Autodesk Inventor part; units mm, degrees
ref_plane "Work Plane1" through (0, 4, 0) normal (0, 1, 0) x (-1, 0, 0)
ref_plane "Work Plane2" through (39, 0, -45) normal (1, 0, 0) x (0, 0, -1)
ref_plane "YZ Plane" through (0, 0, 0) normal (1, 0, 0) x (0, 1, 0)
sketch "Sketch1" plane through (0, 0, 0) normal (0, 1, 0) x (-1, 0, 0)
  line L0 (-10, 0) -> (-63, 0)
  line L1 (-73, -10) -> (-73, -57)
  line L2 (0, -57) -> (0, -10)
  line L3 (-22.5, -57) -> (-22.5, -65)
  line L4 (-22.5, -65) -> (-30, -65)
  line L5 (-30, -65) -> (-30, -57)
  line L6 (-48, -57) -> (-48, -65)
  line L7 (-48, -65) -> (-55.5, -65)
  line L8 (-55.5, -65) -> (-55.5, -57)
  line L9 (-73, -57) -> (-55.5, -57)
  line L10 (-22.5, -57) -> (0, -57)
  line L11 (-37.25, -57) -> (-37.25, -53)
  line L12 (-37.25, -53) -> (-36, -53)
  line L13 (-36, -53) -> (-36, -50)
  line L14 (-36, -50) -> (-37.25, -50)
  line L15 (-37.25, -50) -> (-37.25, -45)
  line L16 (-37.25, -45) -> (-40.75, -45)
  line L17 (-40.75, -45) -> (-40.75, -50)
  line L18 (-40.75, -50) -> (-42, -50)
  line L19 (-42, -50) -> (-42, -53)
  line L20 (-42, -53) -> (-40.75, -53)
  line L21 (-40.75, -53) -> (-40.75, -57)
  line L22 (-48, -57) -> (-40.75, -57)
  line L23 (-37.25, -57) -> (-30, -57)
  arc A0 (0, -10) -> (-10, 0) centre (-10, -10) ccw
  arc A1 (-63, 0) -> (-73, -10) centre (-63, -10) ccw
  line L24 (-5, -17) -> (-10, -17)
  line L25 (-10, -17) -> (-10, -27)
  line L26 (-10, -27) -> (-5, -27)
  line L27 (-5, -27) -> (-5, -17)
  line L28 (-5, -36.5) -> (-10, -36.5)
  line L29 (-10, -36.5) -> (-10, -46.5)
  line L30 (-10, -46.5) -> (-5, -46.5)
  line L31 (-5, -46.5) -> (-5, -36.5)
  line L32 (-63, -17) -> (-68, -17)
  line L33 (-68, -17) -> (-68, -27)
  line L34 (-68, -27) -> (-63, -27)
  line L35 (-63, -27) -> (-63, -17)
  line L36 (-63, -36.5) -> (-68, -36.5)
  line L37 (-68, -36.5) -> (-68, -46.5)
  line L38 (-68, -46.5) -> (-63, -46.5)
  line L39 (-63, -46.5) -> (-63, -36.5)
  line L40 (-39, -45) -> (-39, -65) construction
  point P0 (0, 0)
  point P1 (-73, 0)
  dimension "d0" = 73
  dimension "d1" = 57
  dimension "d2" = 22.5
  dimension "d3" = 7.5
  dimension "d4" = 8
  dimension "d5" = 17.5
  dimension "d6" = 18
  dimension "d7" = 3.5
  dimension "d8" = 6
  dimension "d9" = 4
  dimension "d10" = 3
  dimension "d11" = 5
  dimension "d12" = 10
  dimension "d13" = 5
  dimension "d14" = 10
  dimension "d15" = 5
  dimension "d17" = 9.5
  dimension "d18" = 5
  dimension "d19" = 10.5
extrude "Extrusion1" add sketch "Sketch1" along normal blind 8
sketch "Sketch2" plane through (0, 8, 0) normal (0, 1, 0) x (1, 0, 0)
  line L0 (63, 36.5) -> (63, 46.5) construction
  line L1 (63, 46.5) -> (68, 46.5) construction
  line L2 (68, 46.5) -> (68, 36.5) construction
  line L3 (68, 36.5) -> (63, 36.5) construction
  line L4 (63, 17) -> (63, 27) construction
  line L5 (63, 27) -> (68, 27) construction
  line L6 (68, 27) -> (68, 17) construction
  line L7 (68, 17) -> (63, 17) construction
  line L8 (5, 36.5) -> (5, 46.5) construction
  line L9 (5, 46.5) -> (10, 46.5) construction
  line L10 (10, 46.5) -> (10, 36.5) construction
  line L11 (10, 36.5) -> (5, 36.5) construction
  line L12 (5, 17) -> (5, 27) construction
  line L13 (5, 27) -> (10, 27) construction
  line L14 (10, 27) -> (10, 17) construction
  line L15 (10, 17) -> (5, 17) construction
  line L16 (73, 10) -> (73, 57) construction
  line L17 (73, 57) -> (55.5, 57) construction
  line L18 (55.5, 57) -> (55.5, 65) construction
  line L19 (55.5, 65) -> (48, 65) construction
  line L20 (48, 65) -> (48, 57) construction
  line L21 (48, 57) -> (40.75, 57) construction
  line L22 (40.75, 57) -> (40.75, 53) construction
  line L23 (40.75, 53) -> (42, 53) construction
  line L24 (42, 53) -> (42, 50) construction
  line L25 (42, 50) -> (40.75, 50) construction
  line L26 (40.75, 50) -> (40.75, 45) construction
  line L27 (40.75, 45) -> (37.25, 45) construction
  line L28 (37.25, 45) -> (37.25, 50) construction
  line L29 (37.25, 50) -> (36, 50) construction
  line L30 (36, 50) -> (36, 53) construction
  line L31 (36, 53) -> (37.25, 53) construction
  line L32 (37.25, 53) -> (37.25, 57) construction
  line L33 (37.25, 57) -> (30, 57) construction
  line L34 (30, 57) -> (30, 65) construction
  line L35 (30, 65) -> (22.5, 65) construction
  line L36 (22.5, 65) -> (22.5, 57) construction
  line L37 (22.5, 57) -> (0, 57) construction
  line L38 (0, 57) -> (0, 10) construction
  arc A0 (0, 10) -> (10, 0) centre (10, 10) ccw construction
  line L39 (10, 0) -> (63, 0) construction
  arc A1 (63, 0) -> (73, 10) centre (63, 10) ccw construction
  line L40 (10, 27) -> (5, 27) construction
  line L41 (7.5, 27) -> (7.5, 36.5) construction
  line L42 (5, 36.5) -> (10, 36.5) construction
  line L43 (65.5, 27) -> (65.5, 36.5) construction
  line L44 (68, 36.5) -> (63, 36.5) construction
  line L45 (23.5, 38) -> (54.5, 38) construction
  line L46 (54.5, 38) -> (54.5, 7) construction
  line L47 (54.5, 7) -> (23.5, 7) construction
  line L48 (23.5, 7) -> (23.5, 38) construction
  line L49 (23.5, 22.5) -> (54.5, 22.5) construction
  point P0 (0, 0)
  point P1 (7.5, 31.75)
  point P2 (65.5, 31.75)
  point P3 (17, 22)
  point P4 (39, 22.5)
  dimension "d22" = 31
  dimension "d23" = 31
  dimension "d24" = 7
  dimension "d25" = 23.5
  dimension "d26" = 17
  dimension "d27" = 22
hole "Hole1" at (7.5, 8, -31.75) at (65.5, 8, -31.75) at (23.5, 8, -38) at (54.5, 8, -38) at (54.5, 8, -7) at (23.5, 8, -7) direction (0, -1, 0) diameter 3.5 end through all
hole "Hole2" at (17, 8, -22) direction (0, -1, 0) diameter 8 end through all
hole "Hole3" at (39, 8, -22.5) direction (0, -1, 0) diameter 23 end through all
ref_plane "Work Plane1" through (0, 4, 0) normal (0, 1, 0) x (-1, 0, 0)
ref_plane "Work Plane2" through (39, 0, -45) normal (1, 0, 0) x (0, 0, -1)
equation "\"d49\" = 0.5 * THICKNESS"
properties part number "A8-0002"
CAD build for the part. Positions are in the model's coordinates, mm. A direction names the side the tool comes from. Round coordinates to 2 decimals unless told otherwise and drop trailing zeros. Write each loop counter-clockwise with the first axis right and the second up, starting at its lowest first coordinate (ties: lowest second). Pieces come first, ordered by that corner, then holes. Notation, with made-up numbers: M 45.25,58 L 83.25,58 A23 cw 83.25,85 Z; hole C 65,11 d9. An arc over 180 degrees is marked long. Use a Markdown table: item, result. Add a question column.
1. Slice it at C-C on z = -31.75. Give the cut face in (x, y).
2. Drill centre lines: probe 1 along X at (y, z) = (3.5, -38); probe 2 along X at (y, z) = (7.5, -40); probe 3 along Z at (x, y) = (17, 3.5). Where is each one in solid material? Low to high.
3. Pull direction X, two halves, no side cores. Call faces 1 (the face through (49.2, 3.94, -17.19)), 2 (the face through (52, 4, -65)), 3 (the face through (55.5, 4, -61)): released by +X, released by -X, zero draft, split by the parting line, or undercut.
4. Slice it at D-D on x = 65.5. Give the cut face in (y, z), then the cut area to 3 significant figures.
5. Slice it at A-A on x = 23.5. Give the cut face in (y, z), then the cut area to 3 significant figures.
6. Flat gauge pins, fed straight in: P1, Ø2.5, axis at y = 4.5, z = -62.5, coming from the +X side; P2, Ø3, axis at x = 60.5, y = 7, coming from the -Z side; P3, Ø3, axis at x = 23.5, z = -38, coming from the +Y side. Where does each tip first touch, or does it go through?
7. Slice it at B-B on z = -22.5. Give the cut face in (x, y), then the cut area to 3 significant figures.
8. 3-axis set-ups, long thin cutter, end or side, ignore diameter. For faces 4 (the face through (29, 0, -32)), 5 (the face through (30, 4, -61)), 6 (the face through (63, 4, -22)): which of +Z, -Z, +X, -X, +Y, -Y reach the whole face in a straight line?
Reply:
| question | item | result |
|---|---|---|
| 1 | outline | M 0,0 L 5.75,0 L 5.75,8 L 0,8 Z; M 9.25,0 L 32.17,0 L 32.17,8 L 9.25,8 Z; M 45.83,0 L 63.75,0 L 63.75,8 L 45.83,8 Z; M 67.25,0 L 73,0 L 73,8 L 67.25,8 Z |
| 2 | probe 1 | x = 0 to 5, 10 to 21.75, 25.25 to 52.75, 56.25 to 63, 68 to 73 |
| 2 | probe 2 | x = 0 to 5, 10 to 63, 68 to 73 |
| 2 | probe 3 | z = -57 to -26, -18 to 0 |
| 3 | face 1 | undercut |
| 3 | face 2 | zero draft |
| 3 | face 3 | released by +X |
| 4 | outline | M 0,-57 L 8,-57 L 8,-46.5 L 0,-46.5 Z; M 0,-36.5 L 8,-36.5 L 8,-33.5 L 0,-33.5 Z; M 0,-30 L 8,-30 L 8,-27 L 0,-27 Z; M 0,-17 L 8,-17 L 8,-0.32 L 0,-0.32 Z |
| 4 | area | 265 mm^2 |
| 5 | outline | M 0,-65 L 8,-65 L 8,-39.75 L 0,-39.75 Z; M 0,-36.25 L 8,-36.25 L 8,-8.75 L 0,-8.75 Z; M 0,-5.25 L 8,-5.25 L 8,0 L 0,0 Z |
| 5 | area | 464 mm^2 |
| 6 | P1 | stops at x = 55.5 |
| 6 | P2 | stops at z = -57 |
| 6 | P3 | passes through |
| 7 | outline | M 0,0 L 5,0 L 5,8 L 0,8 Z; M 10,0 L 13.03,0 L 13.03,8 L 10,8 Z; M 20.97,0 L 27.5,0 L 27.5,8 L 20.97,8 Z; M 50.5,0 L 63,0 L 63,8 L 50.5,8 Z; M 68,0 L 73,0 L 73,8 L 68,8 Z |
| 7 | area | 257 mm^2 |
| 8 | face 4 | +Z, -Z, +X, -X, -Y |
| 8 | face 5 | -Z, +Y, -Y |
| 8 | face 6 | +Y, -Y |
